Verification items for the finished model (mm, model axes). Coordinates: 2 decimals unless noted, no trailing zeros. Loops run counter-clockwise (first coordinate to the right, second up) from the corner with the lowest first, then second, coordinate; pieces in that order, holes last. Notation, with made-up numbers: (7.25, 43.25) - (17.25, 43.25) arc R17 ccw to (17.25, 59.25) - close; hole circle Ø7 at (28, -9.5). An arc over 180 degrees is marked (long way). Answer as CSV lines item,"result". Start each with the question number.
1. Cross-section at B-B (y = 2.3). State how many separate pieces and enclosed holes the cut face has, plus the area to 3 significant figures.
2. Material ranges on line 1 (Z direction, x = 11, y = 0.1); line 2 (Z direction, x = 10.5, y = 1.6); line 3 (X direction, y = 1, z = 159), recorded low to high. Write a range as [from, to].
3. Gauge pin test, flat ends, axial feed: P1, Ø1.6, axis at y = 1.5, z = 153.5, coming from the +X side; P2, Ø1.6, axis at y = 1, z = -2, coming from the -X side. Record the tip position at first contact, or that the pin passes through.
4. Cross-section at C-C (z = -34). Enter the section's corners in (x, y) (3 decimals), plus the area to 3 significant figures.
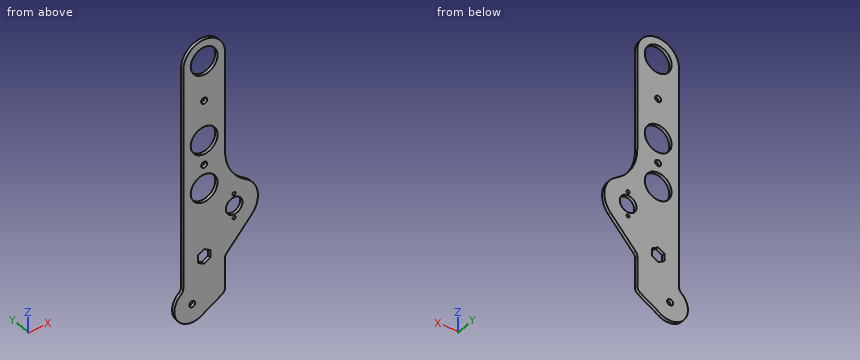
```python
from build123d import *

# Parameters (mm, degrees)
SKETCH1_R           = 14.2875
SKETCH1_R_2         = 3.175
SKETCH1_R_3         = 8.89
SKETCH1_R_4         = 1.650000002
BOSS_EXTRUDE1_DEPTH = 3.175


with BuildPart() as part:
    # Sketch1 → Boss-Extrude1 (new body)
    with BuildSketch(Plane(origin=(0, 0, 0), x_dir=(1, 0, 0), z_dir=(0, 1, 0))):
        with BuildLine():
            Line((0, 24.166221867), (0, -203.2))
            ThreePointArc((0, -203.2), (22.225, -225.425), (44.45, -203.2))
            Line((44.45, -203.2), (44.45, -99.857166641))
            ThreePointArc((44.45, -99.857166641), (50.459229894, -77.430415362), (66.876751279, -61.012893977))
            ThreePointArc((66.876751279, -61.012893977), (79.295297798, -42.786607364), (72.775737997, -21.717360549))
            Line((72.775737997, -21.717360549), (46.15025332, 6.909825302))
            ThreePointArc((46.15025332, 6.909825302), (44.890330322, 8.911022224), (44.45, 11.234447345))
            Line((44.45, 11.234447345), (44.45, 42.161003408))
            ThreePointArc((44.45, 42.161003408), (43.599261314, 45.336003408), (41.275, 47.660264722))
            Line((41.275, 47.660264722), (19.05, 60.491874454))
            ThreePointArc((19.05, 60.491874454), (-6.204468975, 54.74054601), (-2.38125, 29.123189029))
            ThreePointArc((-2.38125, 29.123189029), (-0.62618735, 26.915852524), (0, 24.166221867))
        make_face()
        with Locations(Location((22.225, -203.2, 0), (0, 0, 270))):
            Circle(SKETCH1_R, mode=Mode.SUBTRACT)
        with Locations(Location((22.225, -120.65, 0), (0, 0, 270))):
            Circle(SKETCH1_R, mode=Mode.SUBTRACT)
        with Locations(Location((22.225, -70.9676, 0), (0, 0, 270))):
            Circle(SKETCH1_R, mode=Mode.SUBTRACT)
        with Locations(Location((22.225, -95.25, 0), (0, 0, 270))):
            Circle(SKETCH1_R_2, mode=Mode.SUBTRACT)
        with Locations(Location((22.225, -161.925, 0), (0, 0, 270))):
            Circle(SKETCH1_R_2, mode=Mode.SUBTRACT)
        with Locations(Location((9.525, 43.994090512, 0), (0, 0, 270))):
            Circle(SKETCH1_R_2, mode=Mode.SUBTRACT)
        with Locations(Location((54.176751279, -39.015848721, 0), (0, 0, 270))):
            Circle(SKETCH1_R_3, mode=Mode.SUBTRACT)
        with Locations(Location((54.176751279, -51.515848613, 0), (0, 0, 270))):
            Circle(SKETCH1_R_4, mode=Mode.SUBTRACT)
        with Locations(Location((54.176751279, -26.515848829, 0), (0, 0, 270))):
            Circle(SKETCH1_R_4, mode=Mode.SUBTRACT)
        Polygon((22.225, -7.625642355), (28.829, -3.812821178), (28.829, 3.812821178), (22.225, 7.625642355), (15.621, 3.812821178), (15.621, -3.812821178), align=None, mode=Mode.SUBTRACT)
    extrude(amount=BOSS_EXTRUDE1_DEPTH)


solid = part.part
```
Values follow:
1,separate pieces,"1"
1,enclosed holes,"10"
1,area,"12,100 mm²"
2,line 1,"z = [-62.99, -46.81], [-41.18, 62.13], [79.81, 111.81], [129.49, 194.36], [212.04, 222.38]"
2,line 2,"z = [-63.02, -47.02], [-40.97, 62.8], [79.13, 112.49], [128.81, 195.04], [211.36, 222.08]"
2,line 3,"x = [0, 20.99], [23.46, 44.45]"
3,P1,"stops at x = 44.45"
3,P2,"stops at x = 0"
4,outline,"(-6.693, 0) - (44.45, 0) - (44.45, 3.175) - (-6.693, 3.175) - close"
4,area,"162 mm²"
